Geometry: see drawing. Coordinates: mm, zero at the bounding-box minimum. A direction names the side the tool comes from. Coordinates: 2 decimals unless noted, no trailing zeros. Loops run counter-clockwise (first coordinate to the right, second up) from the corner with the lowest first, then second, coordinate; pieces in that order, holes last. Notation, with made-up numbers: (81, 35.5) -> (128, 35.5) arc R7 cw to (128, 39.5) -> close; hole circle Ø11 at (75, 14.5). An arc over 180 degrees is marked (long way). Put each result on its own line as item: value. Start each with the question number.
1) Set-up query: the marked faces 1 and 2. Return all of +Z, -Z, +X, -X, +Y, -Y with unobstructed straight access to the full face (end or side cutting, diameter ignored); none if empty.
2) Cut plane B-B (x = 15). Return the cut outline in (y, z).
3) Cut plane D-D (x = 8.75). Return the cut outline in (y, z), plus the area to 3 significant figures.
4) Contact query for flat-ended pins moving along their axis: P1, Ø7.5, axis at y = 21.5, z = 4, coming from the -X side; P2, Ø1.5, axis at x = 17.5, z = 26, coming from the +Y side; P3, Ø5, axis at x = 25.5, y = 20, coming from the -Z side. Output: stop coordinate, or through.
5) Cut plane A-A (y = 6). Return the cut outline in (x, z).
6) Material intervals for L1, parallel to Z at x = 15, y = 0.2; L2, parallel to X at y = 0.4, z = 4; L3, parallel to Y at x = 12.5, z = 42.5, sorted ascending.
7) Cut plane C-C (y = 16.25). Return the cut outline in (x, z).
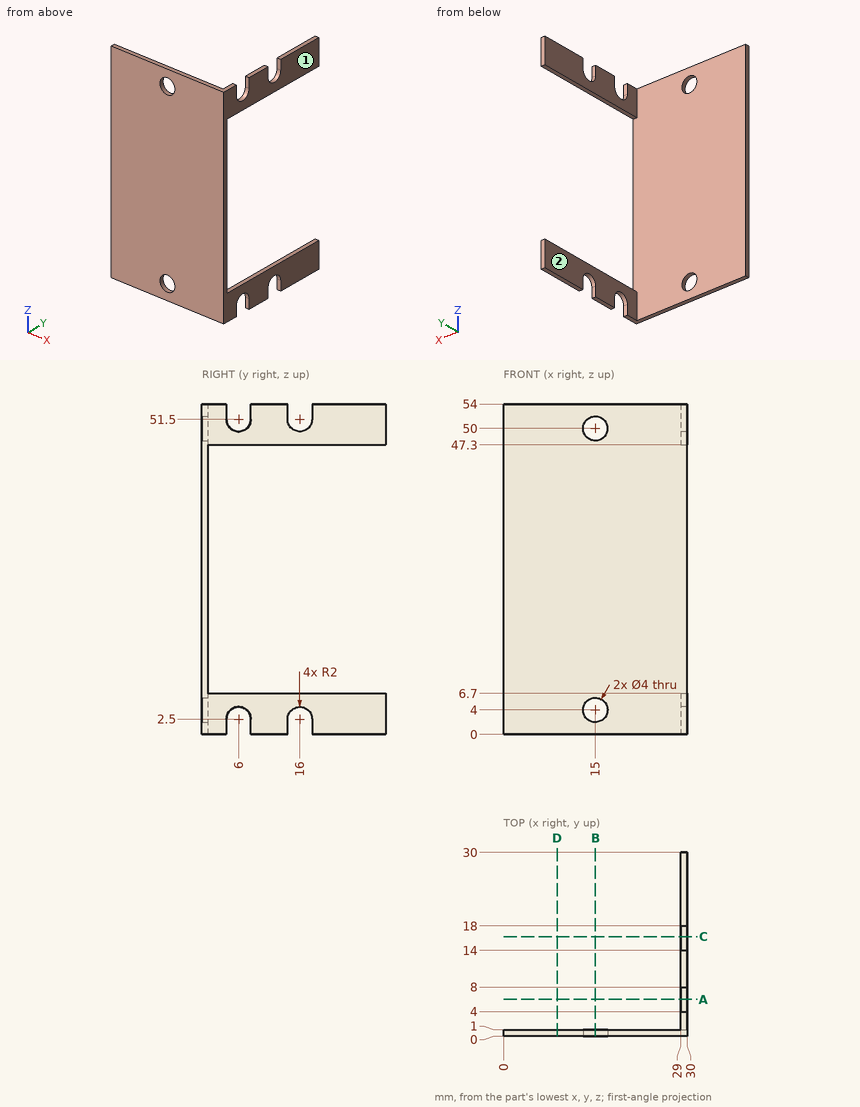
Results found:
1. face 1: +Z, -Z, +X, +Y, -Y
1. face 2: +Z, -Z, -X, +Y
2. outline: (0, 0) -> (1, 0) -> (1, 2) -> (0, 2) -> close; (0, 6) -> (1, 6) -> (1, 48) -> (0, 48) -> close; (0, 52) -> (1, 52) -> (1, 54) -> (0, 54) -> close
3. outline: (0, 0) -> (1, 0) -> (1, 54) -> (0, 54) -> close
3. area: 54.0 mm2
4. P1: stops at x = 29
4. P2: stops at y = 1
4. P3: passes through
5. outline: (29, 4.5) -> (30, 4.5) -> (30, 6.7) -> (29, 6.7) -> close; (29, 47.3) -> (30, 47.3) -> (30, 49.5) -> (29, 49.5) -> close
6. L1: z = 0 to 2, 6 to 48, 52 to 54
6. L2: x = 0 to 13, 17 to 30
6. L3: y = 0 to 1
7. outline: (29, 4.48) -> (30, 4.48) -> (30, 6.7) -> (29, 6.7) -> close; (29, 47.3) -> (30, 47.3) -> (30, 49.52) -> (29, 49.52) -> close
